The listing builds one solid part. Answer for the finished solid, in the listing's coordinates (mm). A direction names the side the tool comes from. Coordinates: 2 decimals unless noted, no trailing zeros. Order: outer loops, then holes, each group sorted by start corner. A loop starts at its lowest first (then second) coordinate and runs counter-clockwise, first axis right, second up.
from build123d import *

# Parameters (mm, degrees)
BOSS_EXTRUDE1_DEPTH = 1900
SKETCH2_R           = 300
CUT_EXTRUDE1_DEPTH  = 2232.591360442
SKETCH4_W           = 250
SKETCH4_H           = 100
CUT_EXTRUDE3_DEPTH  = 550
SHELL1_START        = 320
SHELL1_DEPTH        = 1560
SHELL1_START_2      = 20
SHELL1_2_DEPTH      = 300
SHELL1_3_DEPTH      = 10
BOSS_EXTRUDE2_START = -10
BOSS_EXTRUDE2_DEPTH = 10
BOSS_EXTRUDE3_DEPTH = 10


# Read off the part's stored shape, not the designer's step: Shell1
with BuildPart() as part:
    # Sketch1 → Boss-Extrude1 (new body)
    with BuildSketch(Plane.XY):
        with BuildLine():
            Line((931.575680567, 120), (1100, 120))
            Line((1100, 120), (1100, 0))
            Line((1100, 0), (0, 0))
            Line((0, 0), (0, 120))
            Line((0, 120), (168.424319433, 120))
            ThreePointArc((168.424319433, 120), (550, 400), (931.575680567, 120))
        make_face()
    extrude(amount=BOSS_EXTRUDE1_DEPTH)

    # Sketch2 → Cut-Extrude1 (cut, through all)
    with BuildSketch(Plane.XY.offset(1900)):
        with Locations((550, 0)):
            Circle(SKETCH2_R)
    extrude(amount=-CUT_EXTRUDE1_DEPTH, mode=Mode.SUBTRACT)

    # Sketch4 → Cut-Extrude3 (cut)
    with BuildSketch(Plane(origin=(1100, 0, 0), x_dir=(0, 0, -1), z_dir=(1, 0, 0))):
        with Locations((-175, 50)):
            Rectangle(SKETCH4_W, SKETCH4_H)
    extrude(amount=-CUT_EXTRUDE3_DEPTH, mode=Mode.SUBTRACT)

    # Shell1 outline → Shell1 (cut)
    with BuildSketch(Plane.XY.offset(SHELL1_START)):
        with BuildLine():
            ThreePointArc((916.606055596, 100), (550, 380), (183.393944404, 100))
            Line((183.393944404, 100), (20, 100))
            Line((20, 100), (20, 0))
            Line((20, 0), (250, 0))
            ThreePointArc((250, 0), (550, 300), (850, 0))
            Line((850, 0), (1080, 0))
            Line((1080, 0), (1080, 100))
            Line((1080, 100), (916.606055596, 100))
        make_face()
    extrude(amount=SHELL1_DEPTH, mode=Mode.SUBTRACT)

    # Shell1 2 outline → Shell1 2 (cut)
    with BuildSketch(Plane.XY.offset(SHELL1_START_2)):
        with BuildLine():
            Line((824.954541697, 120), (910.555127546, 120))
            ThreePointArc((910.555127546, 120), (539.552347988, 379.856349911), (183.393944404, 100))
            Line((183.393944404, 100), (20, 100))
            Line((20, 100), (20, 0))
            Line((20, 0), (250, 0))
            ThreePointArc((250, 0), (488.707106893, 293.671893879), (824.954541697, 120))
        make_face()
    extrude(amount=SHELL1_2_DEPTH, mode=Mode.SUBTRACT)

    # Shell1 3 outline → Shell1 3 (cut)
    with BuildSketch(Plane.XY.offset(SHELL1_START_2)):
        with BuildLine():
            ThreePointArc((916.606055596, 100), (913.718086665, 110.041598646), (910.555127546, 120))
            Line((910.555127546, 120), (824.954541697, 120))
            ThreePointArc((824.954541697, 120), (843.671893879, 61.292893107), (850, 0))
            Line((850, 0), (1080, 0))
            Line((1080, 0), (1080, 100))
            Line((1080, 100), (916.606055596, 100))
        make_face()
    extrude(amount=SHELL1_3_DEPTH, mode=Mode.SUBTRACT)

    # Sketch5 → Boss-Extrude2 (add)
    with BuildSketch(Plane(origin=(0, 0, 0), x_dir=(-1, 0, 0), z_dir=(0, 0, -1)).offset(BOSS_EXTRUDE2_START)):
        with BuildLine():
            Line((-850, 0), (-250, 0))
            ThreePointArc((-250, 0), (-550, 300), (-850, 0))
        make_face()
    extrude(amount=BOSS_EXTRUDE2_DEPTH)

    # Sketch6 → Boss-Extrude3 (add)
    with BuildSketch(Plane.XY.offset(1900)):
        with BuildLine():
            Line((850, 0), (250, 0))
            ThreePointArc((250, 0), (550, 300), (850, 0))
        make_face()
    extrude(amount=-BOSS_EXTRUDE3_DEPTH)


solid = part.part
1) Section D-D (y = 190.5) is taken. Give the vertices of the cut face in (x, z), then the cut area to 3 significant figures.
2) Determine the mould class of faces 1 (the face through (103, 100, 937)), 2 (the face through (542.91, 399.937, 936.7)), 3 (the face through (558, 158, 1900)), 4 (the face through (556.597, 299.927, 15.07)) for opening direction Z: released by +Z, released by -Z, zero draft, split by the parting line, or undercut.
3) Section A-A (x = 550) is taken. Give the vertices of the cut face in (y, z), then the cut area to 3 significant figures.
4) Section B-B (z = 741.5) is taken. Give the vertices of the cut face in (x, y).
5) A tool of negligible diameter and unlimited length cuts with its end or side. For faces 5 (the face through (0, 59, 937)), 6 (the face through (999, 100, 1089)), 7 (the face through (968, 100, 177)), from which of +Z, -Z, +X, -X, +Y, -Y can it reach the whole face along a straight path? Write none if from no direction.
6) Consider L1, parallel to Z at x = 861, y = 84; L2, parallel to Z at x = 91, y = 47.5; L3, parallel to X at y = 72, z = 1238.5. Determine where each line is inside the solid, lowest interval first.
7) Each of these flat-tipped pins is pushed along its axis until it touches: P1, Ø8, axis at y = 281, z = 512.5, coming from the +X side; P2, Ø12, axis at x = 435.5, z = 229, coming from the +Y side; P3, Ø5, axis at y = 48.5, z = 26, coming from the -X side; P4, Ø4, axis at y = 191.5, z = 1410.5, coming from the -X side. Where does it stop, or does it pass through?
8) Section C-C (y = 276.5) is taken. Give the vertices of the cut face in (x, z).
Filled sheet:
1. outline: (198.28, 0) - (901.72, 0) - (901.72, 1900) - (198.28, 1900) - close; hole (221.2, 20) - (318.25, 20) - (318.25, 10) - (781.75, 10) - (781.75, 20) - (878.8, 20) - (878.8, 1880) - (781.75, 1880) - (781.75, 1890) - (318.25, 1890) - (318.25, 1880) - (221.2, 1880) - close
1. area: 104,000 mm2
2. face 1: undercut
2. face 2: zero draft
2. face 3: released by +Z
2. face 4: undercut
3. outline: (0, 0) - (400, 0) - (400, 1900) - (0, 1900) - (0, 1890) - (300, 1890) - (300, 1880) - (380, 1880) - (380, 20) - (300, 20) - (300, 10) - (0, 10) - close
3. area: 47,200 mm2
4. outline: (0, 0) - (20, 0) - (20, 100) - (183.39, 100) arc R380 cw to (916.61, 100) - (1080, 100) - (1080, 0) - (1100, 0) - (1100, 120) - (931.58, 120) arc R400 ccw to (168.42, 120) - (0, 120) - close
5. face 5: +Z, -Z, -X, +Y, -Y
5. face 6: -Y
5. face 7: +X, -Y
6. L1: z = 0 to 20, 30 to 50, 300 to 320, 1880 to 1900
6. L2: z = 0 to 20, 1880 to 1900
6. L3: x = 0 to 20, 1080 to 1100
7. P1: stops at x = 838.57
7. P2: stops at y = 385
7. P3: stops at x = 0
7. P4: stops at x = 197.74
8. outline: (260.95, 0) - (839.05, 0) - (839.05, 1900) - (260.95, 1900) - close; hole (289.33, 20) - (433.61, 20) - (433.61, 10) - (666.39, 10) - (666.39, 20) - (810.67, 20) - (810.67, 1880) - (666.39, 1880) - (666.39, 1890) - (433.61, 1890) - (433.61, 1880) - (289.33, 1880) - close
